from build123d import *

# Parameters (mm, degrees)
F1_DEPTH = 50.8
F4_DEPTH = 38.1
F6_DEPTH = 76.2
F9_DEPTH = 38.1


with BuildPart() as f1:
    # F0 (on Front) → F1 (new body)
    with BuildSketch(Plane.XZ):
        Polygon((0, 27.8534215753), (-24.1217706665, -13.9267107877), (24.1217706665, -13.9267107877), align=None)
    extrude(amount=F1_DEPTH)

    # F3 (on Right) → F4 (cut, symmetric)
    with BuildSketch(Plane.YZ):
        Polygon((-4.1414177977, -23.6890129745), (0, -13.9267107877), (-21.6406751424, 0), (-53.4481443465, 0), (-53.4481443465, -20.1891623437), align=None)
    extrude(amount=F4_DEPTH, both=True, mode=Mode.SUBTRACT)

    # F5 (on face) → F6 (cut)
    with BuildSketch(Plane(origin=(-12.0608853333, 0, -20.8900661815), x_dir=(0.8660254038, 0, -0.5), z_dir=(0.5, 0, 0.8660254038))):
        Polygon((0, -21.6406751424), (-13.9267107877, 0), (-23.6785002053, -57.1040175855), (0, -58.6630254984), align=None)
    extrude(amount=F6_DEPTH, mode=Mode.SUBTRACT)

    # F8 (on face) → F9 (cut, symmetric)
    with BuildSketch(Plane(origin=(-4.0202951111, 0, 6.9633553938), x_dir=(0.8660254038, 0, 0.5), z_dir=(0.5, 0, -0.8660254038))):
        Polygon((-6.0183512978, 52.3292906582), (0, 21.6406751424), (13.9267107877, 0), (24.3944823742, 42.0836023986), (17.7801791579, 52.3292906582), align=None)
    extrude(amount=F9_DEPTH, both=True, mode=Mode.SUBTRACT)


solid = f1.part
The listing builds one solid part. Answer for the finished solid, in the listing's coordinates (mm). Give positions to 0.01 mm unless a question says otherwise; leave off trailing zeros. Loops run counter-clockwise (first coordinate to the right, second up) from the corner with the lowest first, then second, coordinate; pieces in that order, holes last. Notation, with made-up numbers: (-35, 74) - (-3, 74) arc R9 cw to (-3, 88) - close; hole circle Ø10 at (87, 27.25). An arc over 180 degrees is marked (long way). Write each question's results on one line, items separated by ' | '.
1. Find section C-C, the plane z = -10. Write down the section's boundary in (x, y), then the cut area to 3 significant figures.
Resolved:
outline: (-21.85, 0) - (-17.32, -6.1) - (17.32, -6.1) - (21.85, 0) - close | area: 239 mm^2
2. Find section B-B, the plane x = -12. Write down the section's boundary in (y, z).
Resolved:
outline: (-10.87, -6.93) - (0, -13.93) - (0, 7.07) - close
3. Find section D-D, the plane z = -5.5. Write down the section's boundary in (x, y).
Resolved:
outline: (-19.26, 0) - (-9.53, -13.09) - (9.53, -13.09) - (19.26, 0) - close
4. Consider probe 1 along Z at (x, y) = (5.5, -2.5); probe 2 along Z at (x, y) = (6, -14); probe 3 along Y at (x, z) = (16, -4). Determine where each line is inside the solid, lowest interval first. Write a range as from..to.
Resolved:
probe 1: z = -12.32..15.11 | probe 2: z = -4.92..-0.56 | probe 3: y = -3.22..0
5. Find section A-A, the plane z = 16. Write down the section's boundary in (x, y), then the cut area to 3 significant figures.
Resolved:
outline: (-6.84, 0) - (0, -9.21) - (6.84, 0) - close | area: 63.0 mm^2
6. Flat-ended cylindrical pins translate along their axes: P1, Ø1.5, axis at x = -14, y = -7, coming from the +Z side; P2, Ø5, axis at x = 3.5, y = -6.5, coming from the -Z side; P3, Ø8, axis at x = 1, y = -5.5, coming from the +Z side. Find the tip coordinate at first contact, or state that the pin passes through.
Resolved:
P1: stops at z = -3.79 | P2: stops at z = -11.35 | P3: stops at z = 25.76
7. For a pull along Z with two mould halves and no side action, classify faces 1 (the face through (-7.455, -8.567, 3.914)), 2 (the face through (0.34, -8.26, -8.61)), 3 (the face through (0, 0, 3)) as +Z half, -Z half, draft (parallel to the pull), parting line (faces both ways), or undercut.
Resolved:
face 1: +Z half | face 2: -Z half | face 3: draft
